```python
from build123d import *

# Parameters (mm, degrees)
F1_DEPTH = 15
F2_R     = 5
F3_DEPTH = 35
F4_R     = 10
F5_DEPTH = 80
F6_R     = 25
F7_DEPTH = 15


with BuildPart() as f1:
    # F0 (on Front) → F1 (new body, symmetric)
    with BuildSketch(Plane.XZ):
        with BuildLine():
            ThreePointArc((81.35, 75), (79.4901280605, 79.4901280605), (75, 81.35))
            Line((75, 81.35), (-75, 81.35))
            ThreePointArc((-75, 81.35), (-79.4901280605, 79.4901280605), (-81.35, 75))
            Line((-81.35, 75), (-81.35, -75))
            ThreePointArc((-81.35, -75), (-79.4901280605, -79.4901280605), (-75, -81.35))
            Line((-75, -81.35), (75, -81.35))
            ThreePointArc((75, -81.35), (79.4901280605, -79.4901280605), (81.35, -75))
            Line((81.35, -75), (81.35, 75))
        make_face()
    extrude(amount=F1_DEPTH, both=True)

    # F2 (on face) → F3 (join)
    with BuildSketch(Plane.XZ.offset(15)):
        Circle(F2_R)
    extrude(amount=F3_DEPTH)

    # F4 (on face) → F5 (join)
    with BuildSketch(Plane(origin=(0, 15, 0), x_dir=(-1, 0, 0), z_dir=(0, 1, 0))):
        Circle(F4_R)
    extrude(amount=F5_DEPTH)

    # F6 (on face) → F7 (join)
    with BuildSketch(Plane(origin=(0, 95, 0), x_dir=(-1, 0, 0), z_dir=(0, 1, 0))):
        Circle(F6_R)
    extrude(amount=F7_DEPTH)


solid = f1.part
```
The listing builds one solid part. Answer for the finished solid, in the listing's coordinates (mm). A direction names the side the tool comes from. Coordinates: 2 decimals unless noted, no trailing zeros. Write each loop counter-clockwise with the first axis right and the second up, starting at its lowest first coordinate (ties: lowest second). Pieces come first, ordered by that corner, then holes. Notation, with made-up numbers: (-0.75, -10) - (50.25, -10) arc R9 cw to (50.25, 0) - close; hole circle Ø7 at (6, 25). An arc over 180 degrees is marked (long way). One line per item, written item: value.
1) Find section B-B (x = 0). Give the vertices of the cut face in (y, z), and give its area (3 significant figures).
Geometry check:
outline: (-50, -5) - (-15, -5) - (-15, -81.35) - (15, -81.35) - (15, -10) - (95, -10) - (95, -25) - (110, -25) - (110, 25) - (95, 25) - (95, 10) - (15, 10) - (15, 81.35) - (-15, 81.35) - (-15, 5) - (-50, 5) - close
area: 7,580 mm2
2) Find section D-D (y = 69). Give the vertices of the cut face in (x, z).
Geometry check:
outline: circle Ø20 at (0, 0)
3) For a pull along Y with two mould halves and no side action, classify faces 1 (the flat face through (0, 95, -11)), 2 (the cylindrical face through (2.17, 54.44, -9.76)), 3 (the flat face through (0, 110, 0)), 4 (the cylindrical face through (-23.846, 102.395, 7.509)) as pulls with the +Y half, pulls with the -Y half, needs draft (parallel to the pull), parting line crosses it, or undercut.
Geometry check:
face 1: undercut
face 2: undercut
face 3: pulls with the +Y half
face 4: needs draft
4) Find section A-A (z = 0). Give the vertices of the cut face in (x, y).
Geometry check:
outline: (-81.35, -15) - (-5, -15) - (-5, -50) - (5, -50) - (5, -15) - (81.35, -15) - (81.35, 15) - (10, 15) - (10, 95) - (25, 95) - (25, 110) - (-25, 110) - (-25, 95) - (-10, 95) - (-10, 15) - (-81.35, 15) - close
5) Find section C-C (z = -16.5). Give the vertices of the cut face in (x, y), and give its area (3 significant figures).
Geometry check:
outline: (-81.35, -15) - (81.35, -15) - (81.35, 15) - (-81.35, 15) - close; (-18.78, 95) - (18.78, 95) - (18.78, 110) - (-18.78, 110) - close
area: 5,440 mm2
6) This flat-tipped pin is pushed along its axis until it touches: pin 1 Ø12 at (x, z) = (34, 30) entering from -Y. Where does it stop, or does it pass through?
Geometry check:
pin 1: stops at y = -15
7) Consider line 1 along Y through (x, z) = (15.5, -11.5); line 2 along Y through (x, z) = (-53, -55); line 3 along Z through (x, y) = (0, 38). Determine where each line is inside the solid, lowest interval first. Write a range as from..to.
Geometry check:
line 1: y = -15..15, 95..110
line 2: y = -15..15
line 3: z = -10..10
8) A tool of negligible diameter and unlimited length cuts with its end or side. For faces 5 (the flat face through (0, -50, 0)), 6 (the cylindrical face through (-1.08, -32.25, -4.88)), from which of +Z, -Z, +X, -X, +Y, -Y can it reach the whole face along a straight path? Write none if from no direction.
Geometry check:
face 5: +Z, -Z, +X, -X, -Y
face 6: -Y
